Design review of the part built by this model. Coordinates are the model's own, in mm. A direction names the side the tool comes from. Give positions to 0.01 mm unless a question says otherwise; leave off trailing zeros. Loops run counter-clockwise (first coordinate to the right, second up) from the corner with the lowest first, then second, coordinate; pieces in that order, holes last. Notation, with made-up numbers: (-4.5, 56.5) - (7.5, 56.5) arc R32 ccw to (7.5, 83.5) - close; hole circle Ø5 at (4.25, 63.5). An arc over 180 degrees is marked (long way). Write each question's results on one line, items separated by ' | '.
Autodesk Inventor part; units mm, degrees
ref_plane "YZ Plane" through (0, 0, 0) normal (1, 0, 0) x (0, 1, 0)
ref_plane "XZ Plane" through (0, 0, 0) normal (0, 1, 0) x (-1, 0, 0)
ref_plane "XY Plane" through (0, 0, 0) normal (0, 0, 1) x (1, 0, 0)
sketch "Sketch1" plane through (0, 0, 0) normal (0, 0, 1) x (1, 0, 0)
  line L0 (-35, 80) -> (35, 80)
  line L1 (35, 80) -> (35, -80)
  line L2 (35, -80) -> (-35, -80)
  line L3 (-35, -80) -> (-35, 80)
  line L4 (-35, 80) -> (35, -80) construction
  line L5 (35, 80) -> (-35, -80) construction
  circle A0 centre (-22.46, 71.46) radius 1.5
  circle A1 centre (22.46, 71.46) radius 1.5
  circle A2 centre (-22.46, -13.46) radius 1.5
  circle A3 centre (22.46, -13.46) radius 1.5
  line L6 (0, 18.5) -> (0, 39.5) construction
  line L7 (-3, 18.5) -> (-3, 39.5)
  line L8 (3, 39.5) -> (3, 18.5)
  arc A4 (-3, 18.5) -> (3, 18.5) centre (0, 18.5) ccw
  arc A5 (3, 39.5) -> (-3, 39.5) centre (0, 39.5) ccw
  line L9 (-11.23, 0) -> (-11.23, 80) construction
  line L10 (-19.46, 18.5) -> (-19.46, 39.5)
  line L11 (-25.46, 39.5) -> (-25.46, 18.5)
  arc A6 (-25.46, 18.5) -> (-19.46, 18.5) centre (-22.46, 18.5) ccw
  arc A7 (-19.46, 39.5) -> (-25.46, 39.5) centre (-22.46, 39.5) ccw
  line L12 (11.23, 5) -> (11.23, 80) construction
  line L13 (25.46, 18.5) -> (25.46, 39.5)
  line L14 (19.46, 39.5) -> (19.46, 18.5)
  arc A8 (19.46, 18.5) -> (25.46, 18.5) centre (22.46, 18.5) ccw
  arc A9 (25.46, 39.5) -> (19.46, 39.5) centre (22.46, 39.5) ccw
  line L15 (-22.46, 62) -> (22.46, 62)
  line L16 (22.46, 62) -> (22.46, 56)
  line L17 (22.46, 56) -> (-22.46, 56)
  line L18 (-22.46, 56) -> (-22.46, 62)
  line L19 (-22.46, 62) -> (22.46, 56) construction
  line L20 (22.46, 62) -> (-22.46, 56) construction
  line L21 (0, 29) -> (-22.46, 29) construction
  line L22 (-22.46, -4) -> (22.46, -4)
  line L23 (22.46, -4) -> (22.46, 2)
  line L24 (22.46, 2) -> (-22.46, 2)
  line L25 (-22.46, 2) -> (-22.46, -4)
  line L26 (0, -22.5) -> (0, -59.5) construction
  line L27 (-3, -22.5) -> (-3, -59.5)
  line L28 (3, -59.5) -> (3, -22.5)
  arc A10 (3, -22.5) -> (-3, -22.5) centre (0, -22.5) ccw
  arc A11 (-3, -59.5) -> (3, -59.5) centre (0, -59.5) ccw
  line L29 (-19.46, -22.5) -> (-19.46, -59.5)
  line L30 (-25.46, -59.5) -> (-25.46, -22.5)
  arc A12 (-19.46, -22.5) -> (-25.46, -22.5) centre (-22.46, -22.5) ccw
  arc A13 (-25.46, -59.5) -> (-19.46, -59.5) centre (-22.46, -59.5) ccw
  line L31 (25.46, -22.5) -> (25.46, -59.5)
  line L32 (19.46, -59.5) -> (19.46, -22.5)
  arc A14 (25.46, -22.5) -> (19.46, -22.5) centre (22.46, -22.5) ccw
  arc A15 (19.46, -59.5) -> (25.46, -59.5) centre (22.46, -59.5) ccw
  point P0 (0, 0)
  point P1 (0, 59)
  point P2 (0, -41)
  dimension "d0" = 3
  dimension "d1" = 22.46
  dimension "d2" = 8.54
  dimension "d5" = 44.92
  dimension "d8" = 84.92
  dimension "d11" = 160
  dimension "d12" = 70
  dimension "d13" = 42.46
  dimension "d14" = 31.96
  dimension "d15" = 22.46
  dimension "d16" = 3
  dimension "d17" = 11.23
  dimension "d18" = 22.46
  dimension "d19" = 44.92
  dimension "d20" = 6
  dimension "d21" = 59
  dimension "d22" = 22.5
  dimension "d23" = 37
  dimension "d24" = 6
  dimension "d25" = 75
  dimension "d26" = 80
  dimension "d27" = 57.46
extrude "Extrusion1" add sketch "Sketch1" against normal blind 10
properties part number "bay_mid"
(1) Wall thickness on line 1 along Y through (x, z) = (4.5, -9); line 2 along X through (y, z) = (38, -8); line 3 along X through (y, z) = (71.46, -7.5): over which ranges is each line inside the solid? List them lowest first. Write a range as from..to.
Answers below:
line 1: -80..-4, 2..56, 62..80 | line 2: -35..-25.46, -19.46..-3, 3..19.46, 25.46..35 | line 3: -35..-23.96, -20.96..20.96, 23.96..35
(2) Take a section at B-B on y = -39. Give the boundary of the cut face in (x, z), plus the area to 3 significant figures.
Answers below:
outline: (-35, -10) - (-25.46, -10) - (-25.46, 0) - (-35, 0) - close; (-19.46, -10) - (-3, -10) - (-3, 0) - (-19.46, 0) - close; (3, -10) - (19.46, -10) - (19.46, 0) - (3, 0) - close; (25.46, -10) - (35, -10) - (35, 0) - (25.46, 0) - close | area: 520 mm2
(3) Take a section at C-C on y = -13.46. Give the boundary of the cut face in (x, z), plus the area to 3 significant figures.
Answers below:
outline: (-35, -10) - (-23.96, -10) - (-23.96, 0) - (-35, 0) - close; (-20.96, -10) - (20.96, -10) - (20.96, 0) - (-20.96, 0) - close; (23.96, -10) - (35, -10) - (35, 0) - (23.96, 0) - close | area: 640 mm2
(4) Draft analysis for pull direction Y (two halves, no side actions). For faces 1 (the flat face through (0, -80, -5)), 2 (the flat face through (0, 62, -5)), 3 (the flat face through (0, 80, -5)), state which applies: pulls with the +Y half, pulls with the -Y half, needs draft (parallel to the pull), parting line crosses it, or undercut.
Answers below:
face 1: pulls with the -Y half | face 2: undercut | face 3: pulls with the +Y half
(5) Take a section at A-A on x = 0. Give the boundary of the cut face in (y, z).
Answers below:
outline: (-80, -10) - (-62.5, -10) - (-62.5, 0) - (-80, 0) - close; (-19.5, -10) - (-4, -10) - (-4, 0) - (-19.5, 0) - close; (2, -10) - (15.5, -10) - (15.5, 0) - (2, 0) - close; (42.5, -10) - (56, -10) - (56, 0) - (42.5, 0) - close; (62, -10) - (80, -10) - (80, 0) - (62, 0) - close
(6) Tool access review of faces 4 (the flat face through (-19.46, 29, -5)), 5 (the flat face through (-35, -1, -5)): name each direction out of +Z, -Z, +X, -X, +Y, -Y from which nothing blocks a thin tool from reaching the whole face with its end or side.
Answers below:
face 4: +Z, -Z | face 5: +Z, -Z, -X, +Y, -Y
(7) Take a section at D-D on z = -5.5. Count the separate pieces of the cut face and the enclosed holes in it, plus the area to 3 significant figures.
Answers below:
separate pieces: 1 | enclosed holes: 12 | area: 9,420 mm2
